from build123d import *

# Parameters (mm, degrees)
SKETCH1_W           = 30
SKETCH1_H           = 8
SKETCH1_R           = 1.5
BOSS_EXTRUDE1_DEPTH = 2
SKETCH2_R           = 1.75
BOSS_EXTRUDE2_DEPTH = 8
SKETCH4_R           = 1.5
CUT_EXTRUDE2_DEPTH  = 18.464249197
FILLET1_R           = 4


with BuildPart() as part:
    # Sketch1 → Boss-Extrude1 (new body)
    with BuildSketch(Plane(origin=(0, 0, 0), x_dir=(1, 0, 0), z_dir=(0, 1, 0))):
        Rectangle(SKETCH1_W, SKETCH1_H)
        with Locations(Location((6, -2, 0), (0, 0, 270))):
            Circle(SKETCH1_R, mode=Mode.SUBTRACT)
    extrude(amount=BOSS_EXTRUDE1_DEPTH)

    # Sketch2 → Boss-Extrude2 (add)
    with BuildSketch(Plane.XY.offset(4)):
        Polygon((-15, 0), (-15, -8), (15, -8), (15, 0), (5, 0), align=None)
        with Locations((-10, -3.5)):
            Circle(SKETCH2_R, mode=Mode.SUBTRACT)
        with Locations((10, -3.5)):
            Circle(SKETCH2_R, mode=Mode.SUBTRACT)
    extrude(amount=-BOSS_EXTRUDE2_DEPTH)

    # Sketch4 → Cut-Extrude2 (cut, through all)
    with BuildSketch(Plane(origin=(0, 0, 0), x_dir=(1, 0, 0), z_dir=(0, 1, 0))):
        with Locations(Location((6, -2, 0), (0, 0, 270))):
            Circle(SKETCH4_R)
    extrude(amount=-CUT_EXTRUDE2_DEPTH, mode=Mode.SUBTRACT)

    # Fillet1
    # the kernel refuses this fillet: 4 mm, written as the material it takes off along each edge
    with BuildSketch(Plane(origin=(-15, -18, -4), x_dir=(1, 0, 0), z_dir=(0, 1, 0)), Plane(origin=(15, 12, -4), x_dir=(-1, 0, 0), z_dir=(0, -1, 0))) as fillet1_piece_1:
        with BuildLine():
            CenterArc((FILLET1_R, -FILLET1_R), FILLET1_R, 90, 90)
            Line((0, -FILLET1_R), (0, 0))
            Line((0, 0), (FILLET1_R, 0))
        make_face()
    extrude(amount=30, mode=Mode.SUBTRACT)


solid = part.part
Part model, mm, in its own coordinate system. Give positions to 0.01 mm unless a question says otherwise; leave off trailing zeros. Order: outer loops, then holes, each group sorted by start corner. A loop starts at its lowest first (then second) coordinate and runs counter-clockwise, first axis right, second up. Notation, with made-up numbers: (41.25, -13) - (48.25, -13) arc R12 ccw to (48.25, 0) - close; hole circle Ø2 at (52, -9). An arc over 180 degrees is marked (long way). Use a Markdown table: item, result.
1) Two-plate mould, pull along X, no slides. Class faces 1 (the cylindrical face through (11.617, -4.17, 0.056)), 2 (the flat face through (0, 2, 0)), 3 (the cylindrical face through (13.797, -2.93, -2.859)): +X half, -X half, draft (parallel to the pull), parting line (faces both ways), or undercut.
Checked values:
| item | result |
|---|---|
| face 1 | undercut |
| face 2 | draft |
| face 3 | +X half |
2) Probe L1, parallel to Y at x = -10, z = -0.25; L2, parallel to X at y = -3.5, z = 1; L3, parallel to X at y = -2.75, z = -1.25. List the from-to ranges inside material, lowest first. Write a range as from..to.
Checked values:
| item | result |
|---|---|
| L1 | -8..-5.25, -1.75..2 |
| L2 | -15..-11.75, -8.25..4.88, 7.12..8.25, 11.75..15 |
| L3 | -14.8..-11.58, -8.42..8.42, 11.58..14.8 |
3) Saw through at B-B on z = 2. List the corners of the cut face in (x, y).
Checked values:
| item | result |
|---|---|
| outline | (-15, -8) - (4.5, -8) - (4.5, 2) - (-15, 2) - close; (7.5, -8) - (15, -8) - (15, 2) - (7.5, 2) - close; hole circle Ø3.5 at (-10, -3.5); hole circle Ø3.5 at (10, -3.5) |
4) Saw through at C-C on y = -7. List the corners of the cut face in (x, z), plus the area to 3 significant figures.
Checked values:
| item | result |
|---|---|
| outline | (-15, 0) arc R4 ccw to (-11, -4) - (11, -4) arc R4 ccw to (15, 0) - (15, 4) - (-15, 4) - close; hole circle Ø3 at (6, 2) |
| area | 226 mm² |
5) Saw through at D-D on y = -2.75. List the corners of the cut face in (x, z), plus the area to 3 significant figures.
Checked values:
| item | result |
|---|---|
| outline | (-15, 0) arc R4 ccw to (-11.58, -3.96) - (-11.58, 4) - (-15, 4) - close; (-8.42, -4) - (8.42, -4) - (8.42, 4) - (-8.42, 4) - close; (11.58, -3.96) arc R4 ccw to (15, 0) - (15, 4) - (11.58, 4) - close; hole circle Ø3 at (6, 2) |
| area | 175 mm² |
6) Flat gauge pins, fed straight in: P1, Ø4.5, axis at x = -10, y = -3.5, coming from the +Z side; P2, Ø1.8, axis at x = 6, z = 2, coming from the +Y side; P3, Ø2, axis at y = -4.5, z = -2, coming from the -X side. Where does each tip first touch, or does it go through?
Checked values:
| item | result |
|---|---|
| P1 | z = 4 |
| P2 | through |
| P3 | x = -14.87 |
7) Saw through at A-A on x = 10. List the corners of the cut face in (y, z), plus the area to 3 significant figures.
Checked values:
| item | result |
|---|---|
| outline | (-8, -4) - (-5.25, -4) - (-5.25, 4) - (-8, 4) - close; (-1.75, -4) - (2, -4) - (2, 4) - (-1.75, 4) - close |
| area | 52.0 mm² |
